Design review of the part built by this model. Coordinates are the model's own, in mm. A direction names the side the tool comes from. Give positions to 0.01 mm unless a question says otherwise; leave off trailing zeros. Loops run counter-clockwise (first coordinate to the right, second up) from the corner with the lowest first, then second, coordinate; pieces in that order, holes last.
Solid Edge part; units mm, degrees
sketch "Sketch1" plane through (0, 0, 0) normal (0, -1, 0) x (1, 0, 0)
  line L0 (-50, -50) -> (50, -50)
  line L1 (50, -50) -> (50, 50)
  line L2 (50, 50) -> (-50, 50)
  line L3 (-50, 50) -> (-50, -50)
  line L4 (45, 45) -> (-45, 45)
  line L5 (-45, 45) -> (-45, -45)
  line L6 (-45, -45) -> (45, -45)
  line L7 (45, -45) -> (45, 45)
extrude "Protrusion1" add sketch "Sketch1" against normal blind 1070
properties part number "1983-1000-002"
Q1. Wall thickness on line 1 (X direction, y = 580.5, z = -29): over which ranges is the line inside the solid? List them lowest first.
Results:
line 1: x = -50 to -45, 45 to 50
Q2. Take a section at B-B (y = 988). Give the boundary of the cut face in (x, z), plus the area to 3 significant figures.
Results:
outline: (-50, -50) - (50, -50) - (50, 50) - (-50, 50) - close; hole (-45, -45) - (45, -45) - (45, 45) - (-45, 45) - close
area: 1,900 mm2
Q3. Draft analysis for pull direction X (two halves, no side actions). For faces 3 (the face through (-50, 528, 1)), 4 (the face through (-48, 0, 4)), 5 (the face through (50, 528, -1)), 6 (the face through (-1, 528, -45)), state which applies: pulls with the +X half, pulls with the -X half, needs draft (parallel to the pull), parting line crosses it, or undercut.
Results:
face 3: pulls with the -X half
face 4: needs draft
face 5: pulls with the +X half
face 6: undercut
Q4. Take a section at C-C (z = -6). Give the boundary of the cut face in (x, y), plus the area to 3 significant figures.
Results:
outline: (-50, 0) - (-45, 0) - (-45, 1070) - (-50, 1070) - close; (45, 0) - (50, 0) - (50, 1070) - (45, 1070) - close
area: 10,700 mm2
Q5. Take a section at A-A (x = 30). Give the boundary of the cut face in (y, z), plus the area to 3 significant figures.
Results:
outline: (0, -50) - (1070, -50) - (1070, -45) - (0, -45) - close; (0, 45) - (1070, 45) - (1070, 50) - (0, 50) - close
area: 10,700 mm2
Q6. Tool access review of faces 1 (the face through (-45, 528, 1)), 2 (the face through (1, 528, 50)): name each direction out of +Z, -Z, +X, -X, +Y, -Y from which nothing blocks a thin tool from reaching the whole face with its end or side.
Results:
face 1: +Y, -Y
face 2: +Z, +X, -X, +Y, -Y
